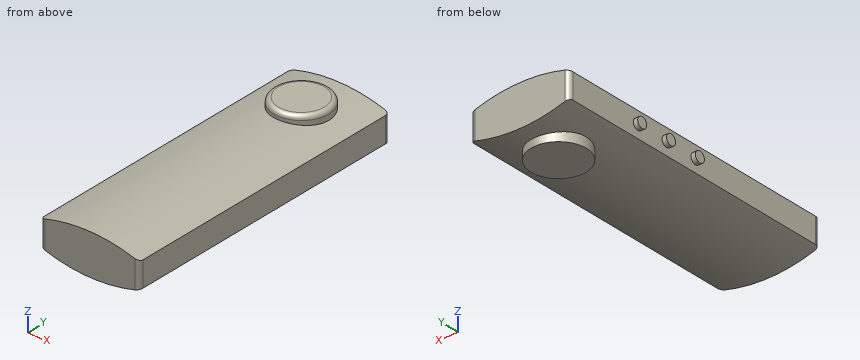
from build123d import *

# Parameters (mm, degrees)
BOSS_EXTRUDE1_DEPTH = 130.12
SKETCH6_R           = 12.3
BOSS_EXTRUDE2_DEPTH = 12.5
SKETCH7_R           = 2.35
BOSS_EXTRUDE3_DEPTH = 2
FILLET1_R           = 2
FILLET2_R           = 2
FILLET3_R           = 2


with BuildPart() as part:
    # Sketch5 → Boss-Extrude1 (new body)
    with BuildSketch(Plane(origin=(0, 0, 0), x_dir=(1, 0, 0), z_dir=(0, 1, 0))):
        with BuildLine():
            Line((-22.1, 5.6), (-22.1, -5.6))
            ThreePointArc((-22.1, -5.6), (0, -9.1), (22.1, -5.6))
            Line((22.1, -5.6), (22.1, 5.6))
            ThreePointArc((22.1, 5.6), (0, 9.1), (-22.1, 5.6))
        make_face()
    extrude(amount=BOSS_EXTRUDE1_DEPTH)

    # Sketch6 → Boss-Extrude2 (add, symmetric)
    with BuildSketch(Plane.XY):
        with Locations(Location((0, 110, 0), (0, 0, 180))):
            Circle(SKETCH6_R)
    extrude(amount=BOSS_EXTRUDE2_DEPTH, both=True)

    # Sketch7 → Boss-Extrude3 (add)
    with BuildSketch(Plane.ZY.offset(22.1)):
        with Locations(Location((0, 94.5, 0), (0, 0, 180))):
            Circle(SKETCH7_R)
        with Locations(Location((0, 79.5, 0), (0, 0, 180))):
            Circle(SKETCH7_R)
        with Locations(Location((0, 64.5, 0), (0, 0, 180))):
            Circle(SKETCH7_R)
    extrude(amount=BOSS_EXTRUDE3_DEPTH)

    # Fillet1
    fillet1_edges = [part.edges().sort_by_distance(p)[0] for p in [
        (12.3, 110, 12.5),
    ]]
    fillet(fillet1_edges, radius=FILLET1_R)

    # Fillet2
    fillet2_edges = [part.edges().sort_by_distance(p)[0] for p in [
        (22.1, 130.12, 0),
        (-22.1, 130.12, 0),
    ]]
    fillet(fillet2_edges, radius=FILLET2_R)

    # Fillet3
    fillet3_edges = [part.edges().sort_by_distance(p)[0] for p in [
        (22.1, 0, 0),
        (-22.1, 0, 0),
    ]]
    fillet(fillet3_edges, radius=FILLET3_R)


solid = part.part
Work out the finished part from the listing and answer in its coordinate system (mm). Give positions to 0.01 mm unless a question says otherwise; leave off trailing zeros. Write each loop counter-clockwise with the first axis right and the second up, starting at its lowest first coordinate (ties: lowest second). Pieces come first, ordered by that corner, then holes. Notation, with made-up numbers: (18, 78) - (66, 78) arc R20 cw to (66, 82) - close; hole circle Ø11 at (44.5, 65). An arc over 180 degrees is marked (long way). One line per item, written item: value. Start each with the question number.
1. Find section A-A (z = 3.5). Write down the section's boundary in (x, y).
2. Find section D-D (y = 56). Write down the section's boundary in (x, z).
3. Consider probe 1 along X at (y, z) = (71, -1); probe 2 along Z at (x, y) = (-20, 41.5); probe 3 along Z at (x, y) = (12, 67). Determine where each line is inside the solid, lowest interval first.
4. Find section C-C (x = 0). Write down the section's boundary in (y, z), then the cut area to 3 significant figures.
5. Find section B-B (y = 79.5). Write down the section's boundary in (x, z), then the cut area to 3 significant figures.
6. Given pin 1 (10 mm diameter, centred on x = -2.5, y = 68, fed in from -Z); pin 2 (8 mm diameter, centred on y = 32.5, z = -0.5, fed in from -X); pin 3 (1 mm diameter, centred on x = 10, y = 99, fed in from -Z), each flat-ended and moving along its own axis, determine where each tip first touches the part or whether it passes through.
Geometry results:
1. outline: (-22.1, 2) arc R2 ccw to (-20.1, 0) - (20.1, 0) arc R2 ccw to (22.1, 2) - (22.1, 128.12) arc R2 ccw to (20.1, 130.12) - (-20.1, 130.12) arc R2 ccw to (-22.1, 128.12) - close
2. outline: (-22.1, -5.6) arc R71.52 ccw to (22.1, -5.6) - (22.1, 5.6) arc R71.52 ccw to (-22.1, 5.6) - close
3. probe 1: -22.1 to 22.1
3. probe 2: -6.25 to 6.25
3. probe 3: -8.09 to 8.09
4. outline: (0, -9.1) - (97.7, -9.1) - (97.7, -12.5) - (122.3, -12.5) - (122.3, -9.1) - (130.12, -9.1) - (130.12, 9.1) - (122.3, 9.1) - (122.3, 10.5) arc R2 ccw to (120.3, 12.5) - (99.7, 12.5) arc R2 ccw to (97.7, 10.5) - (97.7, 9.1) - (0, 9.1) - close
4. area: 2,530 mm2
5. outline: (-24.1, -2.35) - (-22.1, -2.35) - (-22.1, -5.6) arc R71.52 ccw to (22.1, -5.6) - (22.1, 5.6) arc R71.52 ccw to (-22.1, 5.6) - (-22.1, 2.35) - (-24.1, 2.35) - close
5. area: 712 mm2
6. pin 1: z = -9.1
6. pin 2: x = -22.1
6. pin 3: z = -8.47
